Autodesk Inventor part; units mm, degrees
ref_plane "Work Plane1" through (-33.95, 21.7, 2.5) normal (1, 0, 0) x (0, 0, -1)
ref_plane "YZ Plane" through (0, 0, 0) normal (1, 0, 0) x (0, 1, 0)
ref_plane "XZ Plane" through (0, 0, 0) normal (0, 1, 0) x (-1, 0, 0)
sketch "Sketch1" plane through (0, 0, 0) normal (0, 1, 0) x (-1, 0, 0)
  line L0 (0, 0) -> (67.9, 0)
  line L1 (67.9, 0) -> (67.9, -56.3)
  line L2 (67.9, -56.3) -> (0, -56.3)
  line L3 (0, -56.3) -> (0, 0)
  dimension "d4" = 67.9
  dimension "d5" = 56.3
extrude "Extrusion1" add sketch "Sketch1" along normal blind 2
sketch "Sketch4" plane through (0, 0, 0) normal (0, -1, 0) x (1, 0, 0)
  line L0 (2.5, 2.5) -> (-70.4, 2.5)
  line L1 (-70.4, 2.5) -> (-70.4, -58.8)
  line L2 (-70.4, -58.8) -> (2.5, -58.8)
  line L3 (2.5, -58.8) -> (2.5, 2.5)
  line L4 (0, -56.3) -> (0, 0)
  line L5 (0, 0) -> (-67.9, 0)
  line L6 (-67.9, -56.3) -> (0, -56.3)
  line L7 (-67.9, -56.3) -> (-67.9, 0)
  line L8 (0, 0) -> (-67.9, 0)
  line L9 (-67.9, 0) -> (-67.9, -56.3)
  line L10 (-67.9, -56.3) -> (0, -56.3)
  line L11 (0, -56.3) -> (0, 0)
  point P0 (-67.7799, -40.4535)
  point P1 (-67.7799, -17.6706)
  dimension "d35" = 2.5
  dimension "d36" = 2.5
  dimension "d37" = 2.5
  dimension "d38" = 2.5
extrude "Extrusion3" add sketch "Sketch4" against normal blind 21.7
sketch "Sketch5" plane through (2.5, 0, -58.8) normal (0, 0, -1) x (-1, 0, 0)
  line L0 (0, 0) -> (0, -5.5)
  line L1 (0, 0) -> (35.56, 0)
  line L2 (0, 0) -> (72.9, 0)
  arc A0 (35.56, 0) -> (0, -5.5) centre (35.56, -117.7058) ccw
  line L3 (72.9, 0) -> (0, 0)
  point P0 (2.5, 0)
  dimension "d41" = 5.5
  dimension "d42" = 35.56
extrude "Extrusion4" add sketch "Sketch5" against normal up to surface (61.3 mm away)
ref_plane "Work Plane1" through (-33.95, 21.7, 2.5) normal (1, 0, 0) x (0, 0, -1)
mirror "Mirror1" about plane through (-33.95, 21.7, 2.5) normal (1, 0, 0) of "Extrusion4"
sketch "Sketch11" plane through (0, 2, 0) normal (0, 1, 0) x (1, 0, 0)
  line L0 (-67.9, 0) -> (0, 0)
  line L1 (0, 0) -> (0, 56.3)
  line L2 (0, 56.3) -> (-67.9, 56.3)
  line L3 (-67.9, 56.3) -> (-67.9, 0)
  line L4 (-67.9, 0) -> (-52.5, 0)
  line L5 (-52.5, 0) -> (-52.5, 10.9)
  line L6 (-52.5, 10.9) -> (-67.9, 10.9)
  line L7 (-67.9, 10.9) -> (-67.9, 0)
  line L8 (-67.9, 56.3) -> (-52.4, 56.3)
  line L9 (-52.4, 56.3) -> (-52.4, 28.9)
  line L10 (-52.4, 28.9) -> (-67.9, 28.9)
  line L11 (-67.9, 28.9) -> (-67.9, 56.3)
  line L12 (0, 0) -> (-16.2, 0)
  line L13 (-16.2, 0) -> (-16.2, 12.4)
  line L14 (-16.2, 12.4) -> (0, 12.4)
  line L15 (0, 12.4) -> (0, 0)
  line L16 (0, 0) -> (0, 56.3)
  line L17 (0, 56.3) -> (-4, 56.3)
  line L18 (-4, 56.3) -> (-4, 29)
  line L19 (-4, 29) -> (0, 29)
  line L20 (0, 29) -> (0, 56.3)
  dimension "d89" = 15.4
  dimension "d90" = 10.9
  dimension "d91" = 15.5
  dimension "d92" = 27.4
  dimension "d93" = 16.2
  dimension "d94" = 12.4
  dimension "d95" = 4
  dimension "d96" = 27.3
extrude "Extrusion7" add sketch "Sketch11" along normal blind 7 contours L3 L6 L5 L0 | L13 L14 L1 L0 | L3 L2 L9 L10 | L19 L18 L2 L1
sketch "Sketch12" plane through (0, 9, 0) normal (0, 1, 0) x (1, 0, 0)
  line L0 (0, 0) -> (-67.9, 0)
  line L1 (-67.9, 0) -> (-67.9, 56.3)
  line L2 (-67.9, 56.3) -> (0, 56.3)
  line L3 (0, 56.3) -> (0, 0)
  point P0 (-62.6, 5.2)
  point P1 (-5.3, 5)
  point P2 (-62.7, 51.3)
  dimension "d99" = 5.2
  dimension "d100" = 5.3
  dimension "d101" = 5.2
  dimension "d102" = 5
  dimension "d103" = 5
  dimension "d104" = 5.3
hole "Hole6" at (-62.6, 9, -5.2) at (-5.3, 9, -5) at (-62.7, 9, -51.3) direction (0, -1, 0) diameter 3.3 depth 9
sketch "Sketch13" plane through (-70.4, 0, 2.5) normal (0, 0, 1) x (1, 0, 0)
  line L0 (17.9, 9) -> (2.5, 9)
  line L1 (70.4, 9) -> (54.2, 9)
  line L2 (20.8, 10.6) -> (29.4, 10.6)
  line L3 (29.4, 10.6) -> (29.4, 21.7)
  line L4 (29.4, 21.7) -> (20.8, 21.7)
  line L5 (20.8, 21.7) -> (20.8, 10.6)
  line L6 (0, 21.7) -> (72.9, 21.7)
  point P0 (70.4, 0)
  point P1 (2.5, 21.7)
  dimension "d112" = 1.6
  dimension "d113" = 18.3
  dimension "d114" = 8.6
extrude "Extrusion8" cut sketch "Sketch13" against normal up to surface (2.5 mm away)
sketch "Sketch14" plane through (-70.4, 0, -58.8) normal (-1, 0, 0) x (0, 0, 1)
  line L0 (5.85, 9) -> (9.15, 9)
  line L1 (29.9, 9) -> (2.5, 9)
  line L2 (29.9, 9) -> (2.5, 9)
  line L3 (58.8, 9) -> (47.9, 9)
  line L4 (51.95, 9) -> (55.25, 9)
  line L5 (58.8, 9) -> (47.9, 9)
  line L6 (58.8, 9) -> (47.9, 9)
  line L7 (30.4, 9) -> (47.4, 9)
  line L8 (47.4, 9) -> (47.4, 3)
  line L9 (47.4, 3) -> (30.4, 3)
  line L10 (30.4, 3) -> (30.4, 9)
  point P0 (58.8, 0)
  dimension "d118" = 11.4
  dimension "d119" = 17
  dimension "d120" = 6
extrude "Extrusion9" cut sketch "Sketch14" against normal up to surface (2.5 mm away)
sketch "Sketch15" plane through (2.5, 0, -58.8) normal (0, 0, -1) x (-1, 0, 0)
  line L0 (63.55, 9) -> (66.85, 9)
  line L1 (70.4, 9) -> (54.9, 9)
  line L2 (70.4, 9) -> (54.9, 9)
  line L3 (6.5, 9) -> (2.5, 9)
  line L4 (6.5, 9) -> (2.5, 9)
  line L5 (50.2, 21.7) -> (50.2, 16)
  line L6 (50.2, 16) -> (42.2, 16)
  line L7 (42.2, 16) -> (42.2, 21.7)
  line L8 (37.34, 0) -> (35.56, 0)
  line L9 (72.9, 21.7) -> (72.9, -5.5)
  line L10 (0, 21.7) -> (72.9, 21.7)
  line L11 (0, 21.7) -> (0, -5.5)
  arc A0 (35.56, 0) -> (0, -5.5) centre (35.56, -117.7058) ccw
  arc A1 (72.9, -5.5) -> (37.34, 0) centre (37.34, -117.7058) ccw
  line L12 (54.9, 2) -> (70.4, 2)
  line L13 (70.4, 2) -> (55, 2)
  line L14 (55, 2) -> (18.7, 2)
  line L15 (18.7, 2) -> (2.5, 2)
  line L16 (2.5, 2) -> (6.5, 2)
  line L17 (6.5, 2) -> (54.9, 2)
  line L18 (6.15, 9) -> (9.45, 9)
  line L19 (2.5, 9) -> (18.7, 9)
  line L20 (2.5, 9) -> (18.7, 9)
  point P0 (2.5, 0)
  dimension "d124" = 39.7
  dimension "d126" = 7
  dimension "d127" = 8
extrude "Extrusion10" cut sketch "Sketch15" against normal up to surface (2.5 mm away) contours L5 L6 L7 L10
sketch "Sketch16" plane through (-70.4, 21.7, -58.8) normal (-1, 0, 0) x (0, 0, 1)
  line L0 (0, -21.7) -> (61.3, -21.7)
  line L1 (0, -27.2) -> (0, -21.7)
  line L2 (61.3, 0) -> (61.3, -27.2)
  line L3 (0, -27.2) -> (61.3, -27.2)
  arc A0 (61.3, -31.2) -> (0, -31.2) centre (30.65, -146.6278) ccw
  line L4 (0, -27.2) -> (61.3, -27.2)
  line L5 (0, -31.2) -> (0, -27.2)
  line L6 (61.3, -27.2) -> (61.3, -31.2)
  point P0 (58.8, -21.7)
  point P1 (30.65, -26.2)
  dimension "d134" = 4
  dimension "d136" = 4
sketch3d "3D Sketch1"
  arc A0 (-70.4, -5.5, -58.8) -> (-34.84, 0, -58.8) centre (-34.84, -117.7058, -58.8) ccw
  line L0 (-34.84, 0, -58.8) -> (-33.06, 0, -58.8)
  arc A1 (-33.06, 0, -58.8) -> (2.5, -5.5, -58.8) centre (-33.06, -117.7058, -58.8) ccw
sweep "Sweep1" add profiles "Sketch16" path "3D Sketch1" contours L3 A0 L5 | L6 A0 L3
sketch "Sketch17" plane through (-70.4, 21.7, -58.8) normal (-1, 0, 0) x (0, 0, 1)
  line L0 (30.4, -12.7) -> (47.4, -12.7)
  line L1 (47.4, -12.7) -> (47.4, -18.7)
  line L2 (47.4, -18.7) -> (30.4, -18.7)
  line L3 (30.4, -18.7) -> (30.4, -12.7)
  line L4 (61.3, 0) -> (61.3, -31.2)
  line L5 (0, 0) -> (61.3, 0)
  line L6 (0, 0) -> (0, -31.2)
  arc A0 (61.3, -31.2) -> (0, -31.2) centre (30.65, -146.6278) ccw
  line L7 (2.5, 0) -> (58.8, 0)
  line L8 (7, 0) -> (20, 0)
  line L9 (20, 0) -> (20, -9)
  line L10 (20, -9) -> (7, -9)
  line L11 (7, -9) -> (7, 0)
  point P0 (58.8, -21.7)
  dimension "d139" = 13
  dimension "d140" = 9
  dimension "d141" = 7
extrude "Extrusion11" cut sketch "Sketch17" against normal up to surface (2.5 mm away) contours L9 L10 L11 L5
sketch "Sketch18" plane through (-67.9, 9, 0) normal (1, 0, 0) x (0, 0, -1)
  line L0 (51.8, 12.7) -> (51.8, 3.7)
  line L1 (51.8, 3.7) -> (38.8, 3.7)
  line L2 (38.8, 3.7) -> (38.8, 12.7)
  line L3 (0, 12.7) -> (38.8, 12.7)
  line L4 (0, 0) -> (0, 12.7)
  line L5 (0, 0) -> (10.9, 0)
  line L6 (10.9, 0) -> (10.9, -7)
  line L7 (28.9, -7) -> (10.9, -7)
  line L8 (28.9, -7) -> (28.9, 0)
  line L9 (28.9, 0) -> (56.3, 0)
  line L10 (56.3, 0) -> (56.3, 12.7)
  line L11 (51.8, 12.7) -> (56.3, 12.7)
  line L12 (11.4, 0) -> (28.4, 0)
  line L13 (28.4, 0) -> (28.4, -6)
  line L14 (28.4, -6) -> (11.4, -6)
  line L15 (11.4, -6) -> (11.4, 0)
  line L16 (10.9, 3.7) -> (45.4, 3.7)
  line L17 (45.4, 3.7) -> (45.4, 1.7)
  line L18 (45.4, 1.7) -> (10.9, 1.7)
  line L19 (10.9, 1.7) -> (10.9, 3.7)
  line L20 (51.8, 3.7) -> (38.8, 3.7)
  line L21 (10.9, 0) -> (10.9, -7)
  point P0 (0, -9)
  dimension "d145" = 1.7
  dimension "d147" = 10.9
properties part number "Base"
Verification items for the finished model (mm, model axes). A direction names the side the tool comes from. Round coordinates to 2 decimals unless told otherwise and drop trailing zeros. Write each question's results on one line, items separated by ' | '.
1) Access from +Z, -Z, +X, -X, +Y, -Y to the whole of each face (thin tool, end or side, straight path). Record for faces 4 (the flat face through (-69, 6, -11.4)), 5 (the flat face through (-60, 9, -43)), 6 (the flat face through (-69, 17, -51.8)), 7 (the flat face through (2.5, 8, -29)), 8 (the flat face through (-49.6, 16, 1)).
Checks:
face 4: -X | face 5: +Y | face 6: -X, +Y | face 7: +Z, -Z, +X, +Y, -Y | face 8: +Z, +Y
2) Mould release check, pull along X, two halves, no side actions. Record for faces 1 (the flat face through (-63, 0, -5)), 2 (the flat face through (-69, 12.7, -45)), 3 (the flat face through (-70.4, 6, -29)): released by +X, released by -X, zero draft, split by the parting line, or undercut.
Checks:
face 1: undercut | face 2: zero draft | face 3: released by -X
3) Scan lines: L1, parallel to X at y = 2.5, z = -5; L2, parallel to Z at x = -5.3, y = 7.25; L3, parallel to Z at x = -62.7, y = 5.25. Record each from-to range of solid material in increasing order. Write a range as from..to.
Checks:
L1: x = -70.4..-64.24, -60.96..-52.5, -16.2..-6.95, -3.65..2.5 | L2: z = -58.8..-56.3, -12.4..-6.65, -3.35..2.5 | L3: z = -58.8..-52.95, -49.65..-28.9, -10.9..-6.85, -3.55..2.5
4) Gauge pin test, flat ends, axial feed: P1, Ø1.2, axis at x = -69, z = -19.5, coming from the -Y side; P2, Ø2, axis at x = -45.5, z = 1.5, coming from the +Y side; P3, Ø3, axis at x = -62.7, z = -51.3, coming from the -Y side; P4, Ø12, axis at x = -60.5, z = -4, coming from the +Y side. Record the tip position at first contact, or that the pin passes through.
Checks:
P1: stops at y = -5.57 | P2: stops at y = 10.6 | P3: stops at y = -6.05 | P4: stops at y = 21.7
